Can you work these out from the drawing? Everything is in mm from the part's minimum corner. A direction names the side the tool comes from. Coordinates: 2 decimals unless noted, no trailing zeros. Write each loop counter-clockwise with the first axis right and the second up, starting at its lowest first coordinate (ties: lowest second). Pieces come first, ordered by that corner, then holes.
(1) Imagine slicing it at C-C, the plane x = 50. List the corners of the cut face in (y, z) for me.
(2) Imagine slicing it at B-B, the plane z = 66. List the corners of the cut face in (x, y) for me.
(3) For pin 1 Ø6 at (x, y) = (13.5, 61) entering from +Z; pin 2 Ø23 at (x, y) = (50, 50) entering from -Z; pin 3 Ø6 at (y, z) = (69.5, 80) entering from +X, each with a flat end and sliding along its axis, tell me the tip position at first contact or that it passes through.
(4) Please list where these lines run through material, in increasing order: probe 1 along Y at (x, z) = (50, 54); probe 2 along Y at (x, z) = (50, 97); probe 3 along Z at (x, y) = (76, 16.5).
(5) Which directions (+Z, -Z, +X, -X, +Y, -Y) give clear straight access to the entire face, cutting with the end or side of a thin tool? Please do the marked faces 1 and 2.
(6) Thinking about a two-plate mould opening in X: for the marked faces 3, 4, 5 and 6, which applies, released by +X, released by -X, zero draft, split by the parting line, or undercut?
(7) Imagine slicing it at D-D, the plane x = 93.5. List the corners of the cut face in (y, z) for me.
(8) Imagine slicing it at A-A, the plane y = 50. List the corners of the cut face in (x, z) for me, plus the area to 3 significant figures.
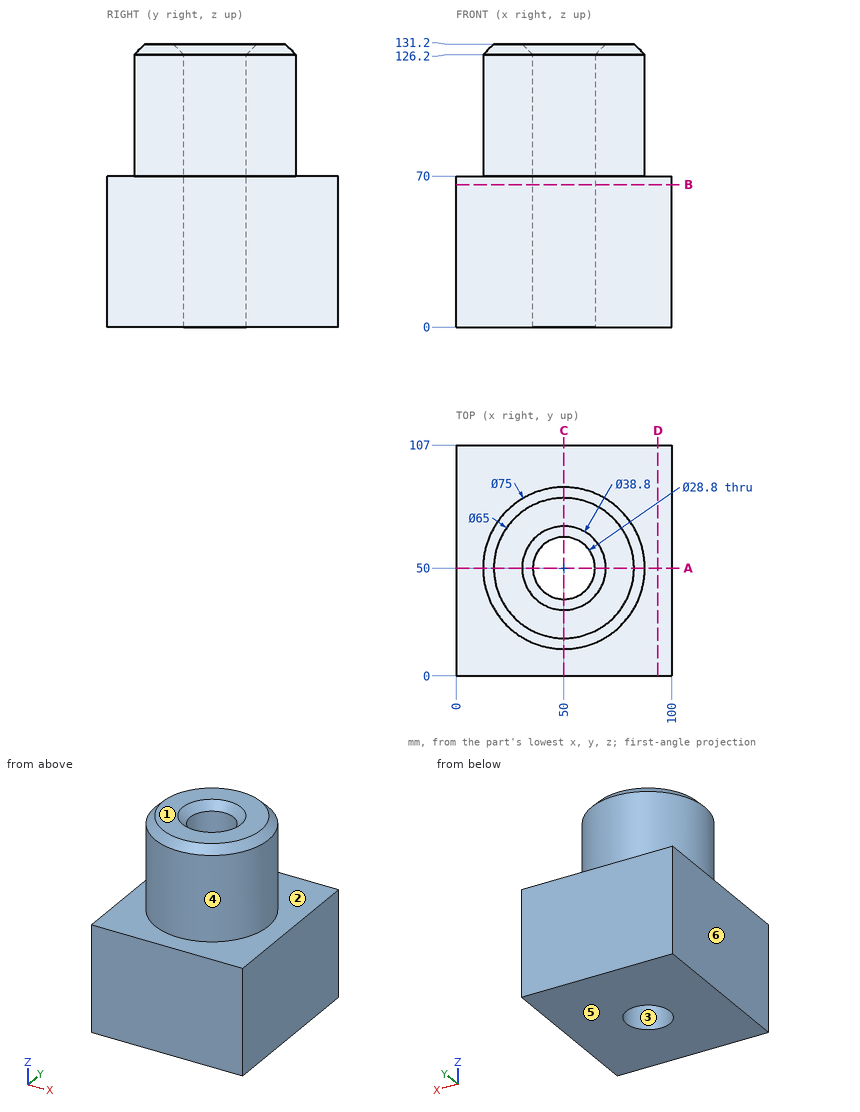
Recorded:
1. outline: (0, 0) - (35.6, 0) - (35.6, 126.2) - (30.6, 131.2) - (17.5, 131.2) - (12.5, 126.2) - (12.5, 70) - (0, 70) - close; (64.4, 0) - (107, 0) - (107, 70) - (87.5, 70) - (87.5, 126.2) - (82.5, 131.2) - (69.4, 131.2) - (64.4, 126.2) - close
2. outline: (0, 0) - (100, 0) - (100, 107) - (0, 107) - close; hole circle Ø28.8 at (50, 50)
3. pin 1: stops at z = 128.58
3. pin 2: passes through
3. pin 3: stops at x = 83.67
4. probe 1: y = 0 to 35.6, 64.4 to 107
4. probe 2: y = 12.5 to 35.6, 64.4 to 87.5
4. probe 3: z = 0 to 70
5. face 1: +Z, +X, -X, +Y, -Y
5. face 2: +Z
6. face 3: undercut
6. face 4: split by the parting line
6. face 5: zero draft
6. face 6: released by -X
7. outline: (0, 0) - (107, 0) - (107, 70) - (0, 70) - close
8. outline: (0, 0) - (35.6, 0) - (35.6, 126.2) - (30.6, 131.2) - (17.5, 131.2) - (12.5, 126.2) - (12.5, 70) - (0, 70) - close; (64.4, 0) - (100, 0) - (100, 70) - (87.5, 70) - (87.5, 126.2) - (82.5, 131.2) - (69.4, 131.2) - (64.4, 126.2) - close
8. area: 7,760 mm2
